CAD build for the part. Positions are in the model's coordinates, mm. A direction names the side the tool comes from. Round coordinates to 2 decimals unless told otherwise and drop trailing zeros. Loops run counter-clockwise (first coordinate to the right, second up) from the corner with the lowest first, then second, coordinate; pieces in that order, holes last. Notation, with made-up numbers: (70.25, -24) - (125.25, -24) arc R3 ccw to (125.25, -20) - close; hole circle Ø6 at (-5.75, 61.25). An arc over 180 degrees is marked (long way). Use one line per item in the form item = value.
from build123d import *

# Parameters (mm, degrees)
F0_R      = 5
F1_DEPTH  = 12
F2_W      = 40
F2_H      = 40
F3_DEPTH  = 6
F4_W      = 40
F4_H      = 12
F5_DEPTH  = 28
F7_DEPTH  = 12
F8_F1_R   = 3
F8_F2_R   = 3
F9_R      = 3
F10_R     = 5
F11_DEPTH = 25


with BuildPart() as f1:
    # F0 (on Front) → F1 (new body)
    with BuildSketch(Plane.XZ):
        with BuildLine():
            Line((40, 20), (-40, 20))
            ThreePointArc((-40, 20), (-47.0710678119, 17.0710678119), (-50, 10))
            Line((-50, 10), (-50, -10))
            ThreePointArc((-50, -10), (-47.0710678119, -17.0710678119), (-40, -20))
            Line((-40, -20), (40, -20))
            ThreePointArc((40, -20), (47.0710678119, -17.0710678119), (50, -10))
            Line((50, -10), (50, 10))
            ThreePointArc((50, 10), (47.0710678119, 17.0710678119), (40, 20))
        make_face()
        with Locations((-35, -10)):
            Circle(F0_R, mode=Mode.SUBTRACT)
        with Locations((35, -10)):
            Circle(F0_R, mode=Mode.SUBTRACT)
    extrude(amount=F1_DEPTH)

    # F2 (on Front) → F3 (cut)
    with BuildSketch(Plane.XZ):
        Rectangle(F2_W, F2_H)
    extrude(amount=F3_DEPTH, mode=Mode.SUBTRACT)

    # F4 (on face) → F5 (join)
    with BuildSketch(Plane.XZ.offset(12)):
        with Locations((0, 14)):
            Rectangle(F4_W, F4_H)
    extrude(amount=F5_DEPTH)

    # F6 (on face) → F7 (join)
    with BuildSketch(Plane.XY.offset(20)):
        with BuildLine():
            Line((20, -40), (-20, -40))
            ThreePointArc((-20, -40), (0, -60), (20, -40))
        make_face()
    extrude(amount=-F7_DEPTH)

    # F8: fillet of radius 3 on 4 edges, made by hand

    # F8_f1
    f8_f1_edges = [f1.edges().sort_by_distance(p)[0] for p in [
        (-20, -26, 8),
        (0, -60, 8),
        (20, -26, 8),
    ]]
    fillet(f8_f1_edges, radius=F8_F1_R)

    # F8_f2
    f8_f2_edges = [f1.edges().sort_by_distance(p)[0] for p in [
        (0, -12, 8),
        (-19.1213203436, -12, 8.8786796564),
        (19.1213203436, -12, 8.8786796564),
    ]]
    fillet(f8_f2_edges, radius=F8_F2_R)

    # F9
    f9_edges = [f1.edges().sort_by_distance(p)[0] for p in [
        (-20, -40, 15.5),
        (0, -60, 11),
        (0, -60, 20),
        (20, -40, 15.5),
        (-31.5, -12, 20),
        (-47.071068, -12, 17.071068),
        (-50, -12, 0),
        (-47.071068, -12, -17.071068),
        (0, -12, -20),
        (47.071068, -12, -17.071068),
        (31.5, -12, 20),
        (50, -12, 0),
        (47.071068, -12, 17.071068),
        (20.87868, -12.87868, 20),
        (20, -27.5, 20),
        (-20, -27.5, 20),
        (-20.87868, -12.87868, 20),
    ]]
    fillet(f9_edges, radius=F9_R)

    # F10 (on face) → F11 (cut)
    with BuildSketch(Plane(origin=(0, 0, 8), x_dir=(1, 0, 0), z_dir=(0, 0, -1))):
        with Locations((0, 40)):
            Circle(F10_R)
    extrude(amount=-F11_DEPTH, mode=Mode.SUBTRACT)


solid = f1.part
1) Drill centre lines: probe 1 along Z at (x, y) = (35, -2); probe 2 along X at (y, z) = (-3.5, -11); probe 3 along Y at (x, z) = (0, 13.75). Where is each one in solid material? Low to high.
Report:
probe_1 = -20 to -15, -5 to 20
probe_2 = -49.95 to -39.9, -30.1 to -20, 20 to 30.1, 39.9 to 49.95
probe_3 = -60 to -45, -35 to -6
2) Slice it at A-A (x = 35). Write the cut outline in (y, z).
Report:
outline = (-12, -17) arc R3 ccw to (-9, -20) - (0, -20) - (0, -15) - (-12, -15) - close; (-12, -5) - (0, -5) - (0, 20) - (-9, 20) arc R3 ccw to (-12, 17) - close
3) Slice it at D-D (x = -27). Write the cut outline in (y, z), plus the area to 3 significant figures.
Report:
outline = (-12, -17) arc R3 ccw to (-9, -20) - (0, -20) - (0, 20) - (-9, 20) arc R3 ccw to (-12, 17) - close
area = 476 mm^2
4) Flat gauge pins, fed straight in: pin 1 (1.5 mm diameter, centred on x = 24.5, z = 3, fed in from -Y); pin 2 (8 mm diameter, centred on x = 35, z = -10, fed in from -Y); pin 3 (3 mm diameter, centred on x = -3, z = 13.5, fed in from -Y); pin 4 (6.5 mm diameter, centred on y = -24.5, z = 15, fed in from +X). Where does each tip first touch, or does it go through?
Report:
pin_1 = -12
pin_2 = through
pin_3 = -59.94
pin_4 = 20
5) Slice it at C-C (z = 2). Write the cut outline in (x, y).
Report:
outline = (-50, -9) arc R3 ccw to (-47, -12) - (47, -12) arc R3 ccw to (50, -9) - (50, 0) - (20, 0) - (20, -6) - (-20, -6) - (-20, 0) - (-50, 0) - close
6) Tool access for faces 1 (the cylindrical face through (-31.38, -11.14, 19.1)), 2 (the cylindrical face through (31.62, -11.14, 19.1)), 3 (the flat face through (-20, -27, 14)): list every direction of +Z, -Z, +X, -X, +Y, -Y with a clear straight run to the whole face (end or side of a thin tool).
Report:
face_1 = +Z, -X, -Y
face_2 = +Z, +X, -Y
face_3 = +Z, -Z, -X, -Y
7) Slice it at B-B (y = -16.5). Write the cut outline in (x, z), plus the area to 3 significant figures.
Report:
outline = (-20, 11) arc R3 ccw to (-17, 8) - (17, 8) arc R3 ccw to (20, 11) - (20, 17) arc R3 ccw to (17, 20) - (-17, 20) arc R3 ccw to (-20, 17) - close
area = 472 mm^2
8) Two-plate mould, pull along X, no slides. Class faces 4 (the cylindrical face through (-20.9, -12.86, 13.96)), 5 (the cylindrical face through (-40, -6, -10)), 6 (the flat face through (20, -27, 14)): +X half, -X half, draft (parallel to the pull), parting line (faces both ways), or undercut.
Report:
face_4 = -X half
face_5 = undercut
face_6 = +X half
